Check sheet for the modelled part. Datum: model origin and axes. Units: mm. Give positions to 0.01 mm unless a question says otherwise; leave off trailing zeros. Write each loop counter-clockwise with the first axis right and the second up, starting at its lowest first coordinate (ties: lowest second). Pieces come first, ordered by that corner, then holes. Notation, with made-up numbers: (54, 31.25) -> (111, 31.25) arc R19 ccw to (111, 39.25) -> close; hole circle Ø6 at (54, 54.5). An arc over 180 degrees is marked (long way). Write each question's results on one line, items separated by ' | '. Start each with the question number.
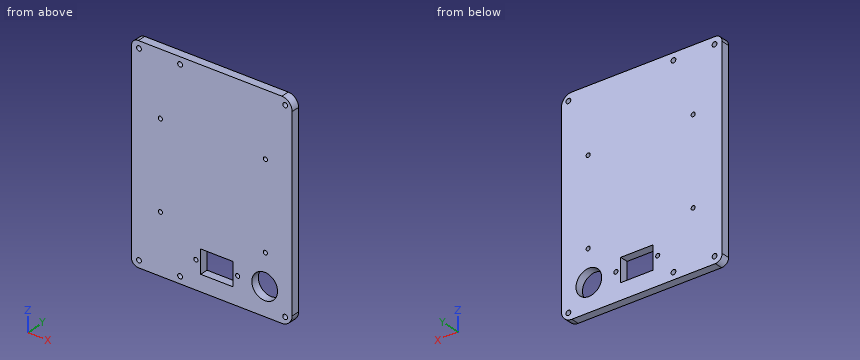
```python
from build123d import *

# Parameters (mm, degrees)
F0_W      = 41
F0_H      = 150.145
F1_DEPTH  = 6
F2_R      = 1.75
F3_DEPTH  = 6.001
F4_W      = 76.25
F4_H      = 150.145
F5_DEPTH  = 6
F6_R      = 5
F7_R      = 7.5
F8_R      = 1.75
F9_DEPTH  = 6.001
F10_R     = 9.375
F10_W     = 23.5
F10_H     = 16.75
F10_R_2   = 1.5
F11_DEPTH = 6.001
F12_R     = 1.5
F13_DEPTH = 6.001


with BuildPart() as f1:
    # F0 (on Front) → F1 (new body)
    with BuildSketch(Plane.XZ):
        Rectangle(F0_W, F0_H)
    extrude(amount=F1_DEPTH)

    # F2 (on face) → F3 (cut, through all)
    with BuildSketch(Plane.XZ.offset(6)):
        with Locations((-15, 70)):
            Circle(F2_R)
        with Locations((15, 70)):
            Circle(F2_R)
        with Locations((-15, -70)):
            Circle(F2_R)
        with Locations((15, -70)):
            Circle(F2_R)
    extrude(amount=-F3_DEPTH, mode=Mode.SUBTRACT)

    # F4 (on face) → F5 (join, through all)
    with BuildSketch(Plane.XZ.offset(6)):
        with Locations((58.625, 0)):
            Rectangle(F4_W, F4_H)
    extrude(amount=-F5_DEPTH)

    # F6
    f6_edges = [f1.edges().sort_by_distance(p)[0] for p in [
        (-20.5, -3, 75.0725),
        (-20.5, -3, -75.0725),
    ]]
    fillet(f6_edges, radius=F6_R)

    # F7
    f7_edges = [f1.edges().sort_by_distance(p)[0] for p in [
        (96.75, -3, 75.0725),
        (96.75, -3, -75.0725),
    ]]
    fillet(f7_edges, radius=F7_R)

    # F8 (on face) → F9 (cut, through all)
    with BuildSketch(Plane.XZ.offset(6)):
        with Locations((91.668, 70)):
            Circle(F8_R)
        with Locations((91.668, -70)):
            Circle(F8_R)
    extrude(amount=-F9_DEPTH, mode=Mode.SUBTRACT)

    # F10 (on face) → F11 (cut, through all)
    with BuildSketch(Plane.XZ.offset(6)):
        with Locations((76.75, -55.0725)):
            Circle(F10_R)
        with Locations((41.75, -55.0725)):
            Rectangle(F10_W, F10_H)
        with Locations((57, -55.0725)):
            Circle(F10_R_2)
        with Locations((26.5, -55.0725)):
            Circle(F10_R_2)
    extrude(amount=-F11_DEPTH, mode=Mode.SUBTRACT)

    # F12 (on face) → F13 (cut, through all)
    with BuildSketch(Plane.XZ.offset(6)):
        with Locations((0.625, -32.5525)):
            Circle(F12_R)
        with Locations((77.225, -32.5525)):
            Circle(F12_R)
        with Locations((0.625, 29.1575)):
            Circle(F12_R)
        with Locations((77.225, 29.1575)):
            Circle(F12_R)
    extrude(amount=-F13_DEPTH, mode=Mode.SUBTRACT)


solid = f1.part
```
Item 1: Section check B-B on y = -1.8. Count the separate pieces of the cut face and the enclosed holes in it, then the cut area to 3 significant figures.
Item 2: Thickness scan on probe 1 along Z at (x, y) = (-15, -4); probe 2 along Z at (x, y) = (76.75, -3.45); probe 3 along Z at (x, y) = (48, -1). Record the ranges inside material, lowest first. Write a range as from..to.
Item 3: Depth check by flat-ended pin: pin 1 Ø4 at (x, z) = (77.22, 29.16) entering from -Y; pin 2 Ø2.5 at (x, z) = (77.22, -32.55) entering from -Y. Enter the tip coordinate at first touch or a pass-through.
Item 4: Section check A-A on x = 15. Record the boundary of the cut face in (y, z).
Check sheet entries:
1) separate pieces: 1 | enclosed holes: 14 | area: 16,800 mm^2
2) probe 1: z = -75.07..-71.75, -68.25..68.25, 71.75..75.07 | probe 2: z = -75.07..-64.45, -45.7..-33.98, -31.13..27.73, 30.58..75.07 | probe 3: z = -75.07..-63.45, -46.7..75.07
3) pin 1: stops at y = -6 | pin 2: passes through
4) outline: (-6, -75.07) -> (0, -75.07) -> (0, -71.75) -> (-6, -71.75) -> close; (-6, -68.25) -> (0, -68.25) -> (0, 68.25) -> (-6, 68.25) -> close; (-6, 71.75) -> (0, 71.75) -> (0, 75.07) -> (-6, 75.07) -> close
